```python
from build123d import *

# Parameters (mm, degrees)
SKETCH1_W                = 179
SKETCH1_H                = 78.998711306
BOSS_EXTRUDE1_DEPTH      = 1
FILLET1_R                = 3
CUT_EXTRUDE1_DEPTH       = 142.273697371
F_7_0_7_DIAMETER_HOLE1_D = 7
LPATTERN1_COUNT          = 3
LPATTERN1_PITCH          = 23.5
LPATTERN1_COPY_1_DEPTH   = 142.273697371
LPATTERN1_COPY_2_DEPTH   = 142.273697371


with BuildPart() as part:
    # Sketch1 → Boss-Extrude1 (new body)
    # profile 1 of 2: a face of its own
    with BuildSketch(Plane.XY):
        with Locations((42, 12.124355653)):
            Rectangle(SKETCH1_W, SKETCH1_H)
        with BuildLine():
            ThreePointArc((-6.75, -4.38634244), (0, -8.05), (6.75, -4.38634244))
            Line((6.75, -4.38634244), (6.75, 4.38634244))
            ThreePointArc((6.75, 4.38634244), (0, 8.05), (-6.75, 4.38634244))
            Line((-6.75, 4.38634244), (-6.75, -4.38634244))
        make_face(mode=Mode.SUBTRACT)
    # profile 2 of 2: a face of its own
    with BuildSketch(Plane.XY):
        with BuildLine():
            Line((-6.75, -4.38634244), (-6.75, 4.38634244))
            ThreePointArc((-6.75, 4.38634244), (0, 8.05), (6.75, 4.38634244))
            Line((6.75, 4.38634244), (6.75, -4.38634244))
            ThreePointArc((6.75, -4.38634244), (0, -8.05), (-6.75, -4.38634244))
        make_face()
    extrude(amount=BOSS_EXTRUDE1_DEPTH)

    # Fillet1
    fillet1_edges = [part.edges().sort_by_distance(p)[0] for p in [
        (-47.5, -27.375, 0.5),
        (-47.5, 51.623711306, 0.5),
        (131.5, 51.623711306, 0.5),
        (131.5, -27.375, 0.5),
    ]]
    fillet(fillet1_edges, radius=FILLET1_R)

    # Sketch4 → Cut-Extrude1 (cut, through all)
    with BuildSketch(Plane.XY.offset(1)):
        with BuildLine():
            Line((113.25, 29.010053746), (113.25, 20.237368866))
            ThreePointArc((113.25, 20.237368866), (106.5, 16.573711306), (99.75, 20.237368866))
            Line((99.75, 20.237368866), (99.75, 29.010053746))
            ThreePointArc((99.75, 29.010053746), (106.5, 32.673711306), (113.25, 29.010053746))
        make_face()
    cut_extrude1 = extrude(amount=-CUT_EXTRUDE1_DEPTH, mode=Mode.SUBTRACT)

    # 7.0 _7_ Diameter Hole1 (through all)
    with Locations(Plane.XY.offset(1)):
        with Locations((42, 44.623711306), (-40.5, 44.623711306), (124.5, 44.623711306), (124.5, -20.375), (45.364988053, -20.375), (-40.5, -20.375)):
            Hole(F_7_0_7_DIAMETER_HOLE1_D / 2)

    # Mirror1: Cut-Extrude1 across plane
    add(cut_extrude1.mirror(Plane.ZX.offset(12.124355653)), mode=Mode.SUBTRACT)

    # LPattern1: Cut-Extrude1 ×3
    with Locations(*[(-i * LPATTERN1_PITCH, 0, 0) for i in range(1, LPATTERN1_COUNT)]):
        add(cut_extrude1, mode=Mode.SUBTRACT)

    # LPattern1 copy 1 sketch → LPattern1 copy 1 (cut, through all)
    with BuildSketch(Plane(origin=(-23.5, 24.248711306, 1), x_dir=(1, 0, 0), z_dir=(0, 0, 1))):
        with BuildLine():
            Line((113.25, -29.010053746), (113.25, -20.237368866))
            ThreePointArc((113.25, -20.237368866), (106.5, -16.573711306), (99.75, -20.237368866))
            Line((99.75, -20.237368866), (99.75, -29.010053746))
            ThreePointArc((99.75, -29.010053746), (106.5, -32.673711306), (113.25, -29.010053746))
        make_face()
    extrude(amount=-LPATTERN1_COPY_1_DEPTH, mode=Mode.SUBTRACT)

    # LPattern1 copy 2 sketch → LPattern1 copy 2 (cut, through all)
    with BuildSketch(Plane(origin=(-47, 24.248711306, 1), x_dir=(1, 0, 0), z_dir=(0, 0, 1))):
        with BuildLine():
            Line((113.25, -29.010053746), (113.25, -20.237368866))
            ThreePointArc((113.25, -20.237368866), (106.5, -16.573711306), (99.75, -20.237368866))
            Line((99.75, -20.237368866), (99.75, -29.010053746))
            ThreePointArc((99.75, -29.010053746), (106.5, -32.673711306), (113.25, -29.010053746))
        make_face()
    extrude(amount=-LPATTERN1_COPY_2_DEPTH, mode=Mode.SUBTRACT)


solid = part.part
```
Can you work these out from the model? Positions are in its coordinate system, mm. A direction names the side the tool comes from. Give positions to 0.01 mm unless a question says otherwise; leave off trailing zeros. Order: outer loops, then holes, each group sorted by start corner. A loop starts at its lowest first (then second) coordinate and runs counter-clockwise, first axis right, second up. Notation, with made-up numbers: (-21, 16.5) - (-15, 16.5) arc R28 cw to (-15, 54.5) - close; hole circle Ø1 at (72, 76). An arc over 180 degrees is marked (long way). Use a Markdown table: item, result. Add a question column.
Q1. If we section it at C-C on x = 58: Write out the boundary of the cut face in (y, z) (3 decimals).
Q2. If we section it at A-A on y = 25.5: Write out the boundary of the cut face in (x, z).
Q3. If we section it at D-D on z = 0.15: Count the separate pieces of the cut face and the enclosed holes in it, plus the area to 3 significant figures.
Q4. If we mould it in two halves opening along Y, with no side actions, what happens to faces 1 (the cylindrical face through (121.162, -19.324, 0.493)), 2 (the cylindrical face through (-46.645, -26.473, 0.507)), 3 (the flat face through (41, 13, 1)), 4 (the cylindrical face through (106.388, 32.673, 0.507))? For each: released by +Y, released by -Y, zero draft, split by the parting line, or undercut.
Q5. If we section it at B-B on x = 124.5: Write out the boundary of the cut face in (y, z) (3 decimals).
Q6. Please list where these lines run through material, in increasing order: line 1 along X through (y, z) = (-2.5, 0.6); line 2 along Y through (x, z) = (-40.5, 0.55) (3 decimals); line 3 along X through (y, z) = (45, 0.95).
Q7. On a 3-axis mill with a long thin cutter (end or side, diameter ignored), from which of +Z, -Z, +X, -X, +Y, -Y can I reach the whole of each face in a straight line? I mean faces 5 (the cylindrical face through (106.612, 16.574, 0.507)), 6 (the cylindrical face through (-46.645, 50.722, 0.507)). Say none if no direction works.
Answers follow:
| question | item | result |
|---|---|---|
| 1 | outline | (-27.375, 0) - (-8.284, 0) - (-8.284, 1) - (-27.375, 1) - close; (7.534, 0) - (16.715, 0) - (16.715, 1) - (7.534, 1) - close; (32.533, 0) - (51.624, 0) - (51.624, 1) - (32.533, 1) - close |
| 2 | outline | (-47.5, 0) - (52.75, 0) - (52.75, 1) - (-47.5, 1) - close; (66.25, 0) - (76.25, 0) - (76.25, 1) - (66.25, 1) - close; (89.75, 0) - (99.75, 0) - (99.75, 1) - (89.75, 1) - close; (113.25, 0) - (131.5, 0) - (131.5, 1) - (113.25, 1) - close |
| 3 | separate pieces | 1 |
| 3 | enclosed holes | 12 |
| 3 | area | 12,800 mm^2 |
| 4 | face 1 | undercut |
| 4 | face 2 | released by -Y |
| 4 | face 3 | zero draft |
| 4 | face 4 | undercut |
| 5 | outline | (-27.375, 0) - (-23.875, 0) - (-23.875, 1) - (-27.375, 1) - close; (-16.875, 0) - (41.124, 0) - (41.124, 1) - (-16.875, 1) - close; (48.124, 0) - (51.624, 0) - (51.624, 1) - (48.124, 1) - close |
| 6 | line 1 | x = -47.5 to 52.75, 66.25 to 76.25, 89.75 to 99.75, 113.25 to 131.5 |
| 6 | line 2 | y = -27.375 to -23.875, -16.875 to 41.124, 48.124 to 51.624 |
| 6 | line 3 | x = -47.5 to -43.98, -37.02 to 38.52, 45.48 to 121.02, 127.98 to 131.5 |
| 7 | face 5 | +Z, -Z |
| 7 | face 6 | +Z, -Z, -X, +Y |
